from build123d import *

# Parameters (mm, degrees)
SKETCH1_R           = 9.525
SHAFT_DEPTH         = 7.62
SKETCH11_R          = 9.779
SKETCH11_R_2        = 8.509
THREAD_RECESS_DEPTH = 1.016
SKETCH13_R          = 7.1374
LARGE_HOLE_DEPTH    = 22.886783683
SKETCH14_R          = 2.413
SMALL_HOLE_DEPTH    = 22.886783683
CHAMFER1_SIZE       = 1.778
SKETCH15_R          = 0.635
TOOL_HOLES_DEPTH    = 1.524


with BuildPart() as part:
    # Sketch1 → Shaft (new body)
    with BuildSketch(Plane(origin=(0, 0, 0), x_dir=(1, 0, 0), z_dir=(0, 1, 0))):
        with Locations(Location((0, 0, 0), (0, 0, 270))):
            Circle(SKETCH1_R)
    extrude(amount=-SHAFT_DEPTH)

    # Sketch11 → Thread Recess (cut)
    with BuildSketch(Plane(origin=(0, 0, 0), x_dir=(1, 0, 0), z_dir=(0, 1, 0))):
        Circle(SKETCH11_R)
        with Locations(Location((0, 0, 0), (0, 0, 270))):
            Circle(SKETCH11_R_2, mode=Mode.SUBTRACT)
    extrude(amount=-THREAD_RECESS_DEPTH, mode=Mode.SUBTRACT)

    # Sketch12 → Standard Connector (revolve)
    with BuildSketch(Plane.XY, mode=Mode.PRIVATE) as standard_connector_sk:
        with BuildLine():
            Line((0, 0), (10.16, 0))
            Line((10.16, 0), (10.16, 1.27))
            ThreePointArc((10.16, 1.27), (9.788025612, 2.168025612), (8.89, 2.54))
            Line((8.89, 2.54), (4.445, 2.54))
            Line((4.445, 2.54), (4.445, 8.509))
            Line((4.445, 8.509), (3.3655, 8.956143541))
            Line((3.3655, 8.956143541), (3.3655, 11.496143541))
            Line((3.3655, 11.496143541), (4.445, 11.943287081))
            Line((4.445, 11.943287081), (4.445, 13.785882072))
            Line((4.445, 13.785882072), (4.0005, 13.97))
            Line((4.0005, 13.97), (4.0005, 16.51))
            Line((4.0005, 16.51), (0, 16.51))
            Line((0, 16.51), (0, 0))
        make_face()
    revolve(standard_connector_sk.sketch.rotate(Axis((0, 0, 0), (0, 1, 0)), 90), axis=Axis((0, 0, 0), (0, 1, 0)))

    # Sketch13 → Large Hole (cut, through all)
    with BuildSketch(Plane(origin=(0, 0, 0), x_dir=(1, 0, 0), z_dir=(0, 1, 0))):
        with Locations(Location((0, 0, 0), (0, 0, 270))):
            Circle(SKETCH13_R)
    extrude(amount=-LARGE_HOLE_DEPTH, mode=Mode.SUBTRACT)

    # Sketch14 → Small Hole (cut, through all)
    with BuildSketch(Plane(origin=(0, 0, 0), x_dir=(1, 0, 0), z_dir=(0, 1, 0))):
        with Locations(Location((0, 0, 0), (0, 0, 270))):
            Circle(SKETCH14_R)
    extrude(amount=SMALL_HOLE_DEPTH, mode=Mode.SUBTRACT)

    # Chamfer1
    chamfer1_edges = [part.edges().sort_by_distance(p)[0] for p in [
        (0, 0, -2.413),
    ]]
    chamfer(chamfer1_edges, length=CHAMFER1_SIZE)

    # Sketch15 → Tool Holes (cut)
    with BuildSketch(Plane(origin=(0, 2.54, 0), x_dir=(-1, 0, 0), z_dir=(0, 1, 0))):
        with Locations(Location((0, -7.62, 0), (0, 0, 90))):
            Circle(SKETCH15_R)
        with Locations(Location((0, 7.62, 0), (0, 0, 270))):
            Circle(SKETCH15_R)
    extrude(amount=-TOOL_HOLES_DEPTH, mode=Mode.SUBTRACT)


solid = part.part
Read the model definition and answer for the solid it produces. Units are mm, in the model's axes. A direction names the side the tool comes from. Coordinates: 2 decimals unless noted, no trailing zeros. Order: outer loops, then holes, each group sorted by start corner. A loop starts at its lowest first (then second) coordinate and runs counter-clockwise, first axis right, second up. Notation, with made-up numbers: (30.5, 71) - (38.5, 71) arc R17 ccw to (38.5, 87) - close; hole circle Ø1 at (-8, 19). An arc over 180 degrees is marked (long way). Use one line per item in the form item = value.
(1) Given pin 1 Ø8 at (x, y) = (-2.5, 9.5) entering from -Z (3 decimals); pin 2 Ø12 at (x, y) = (-5, 6.5) entering from +Z; pin 3 Ø3 at (x, y) = (1, 3) entering from -Z, each flat-ended and moving along its own axis, determine where each tip first touches the part or whether it passes through.
Computed values:
pin_1 = -4.445
pin_2 = 10
pin_3 = -10.11
(2) Straight lines are drawn through the part: L1, parallel to Y at x = -3, z = 8; L2, parallel to Y at x = 0.25, z = -6; L3, parallel to Y at x = 1, z = -4. For each, find the intervals that lie inside material, in ascending order.
Computed values:
L1 = -7.62 to -1.02, 0 to 2.54
L2 = 0 to 2.54
L3 = 0.07 to 8.64, 11.81 to 13.92
(3) Which of the six approach directions +Z, -Z, +X, -X, +Y, -Y give full straight-line access (tool end or side, diameter ignored) to faces 1 (the face through (8.437, -0.501, -1.108)), 2 (the face through (3.9, 15.3, 0.9)), 3 (the face through (-5.796, -4.272, -7.559))?
Computed values:
face_1 = none
face_2 = +Y
face_3 = -Y
(4) Section A-A, the plane y = 5 is taken. Give the vertices of the cut face in (x, z) (3 decimals), then the cut area to 3 significant figures.
Computed values:
outline = circle Ø8.89 at (0, 0); hole circle Ø4.826 at (0, 0)
area = 43.8 mm²
(5) For a pull along Z with two mould halves and no side action, classify faces 4 (the face through (0, 1.016, -8)), 5 (the face through (7.5, 0, 4.5)), 6 (the face through (4.34, 12.88, 0.96)) as pulls with the +Z half, pulls with the -Z half, needs draft (parallel to the pull), parting line crosses it, or undercut.
Computed values:
face_4 = undercut
face_5 = needs draft
face_6 = parting line crosses it
